Source: CAD feature listing. Evaluate the final solid. Frame: model axes, mm. A direction names the side the tool comes from. Round coordinates to 2 decimals unless told otherwise and drop trailing zeros. Loops run counter-clockwise (first coordinate to the right, second up) from the corner with the lowest first, then second, coordinate; pieces in that order, holes last.
(1) Section B-B, the plane x = -11.5. Return the cut outline in (y, z) (3 decimals).
(2) Set-up query: faces 4 (the cylindrical face through (-17.786, 5.966, 2.335)), 5 (the cylindrical face through (-3.36, 0.63, 9.82)). Return all of +Z, -Z, +X, -X, +Y, -Y with unobstructed straight access to the full face (end or side cutting, diameter ignored); none if empty.
(3) Section A-A, the plane z = -10. Return the cut outline in (x, y) (3 decimals).
(4) Mould query, pull axis Y, two halves, no side actions, for faces 1 (the cylindrical face through (-6.38, 5.95, 15.4)), 2 (the flat face through (0, 0, 0)), 3 (the flat face through (20, 1, 0)). Classes: pulls with the +Y half, pulls with the -Y half, needs draft (parallel to the pull), parting line crosses it, or undercut.
(5) Section D-D, the plane z = 15. Count the separate pieces of the cut face and the enclosed holes in it, plus the area to 3 significant figures.
(6) Section C-C, the plane y = 2.25. Return the cut outline in (x, z).
(7) Material intervals for probe 1 along Y at (x, z) = (-18, 7) (3 decimals); probe 2 along Z at (x, y) = (-5.5, 11.5); probe 3 along Z at (x, y) = (0.5, 6), sorted ascending.
```python
from build123d import *

# Parameters (mm, degrees)
SKETCH1_W           = 40
SKETCH1_H           = 40
SKETCH1_R           = 16.66875
SKETCH1_R_2         = 1.905
BOSS_EXTRUDE1_DEPTH = 1.27
SKETCH2_R           = 17.93875
SKETCH2_R_2         = 16.66875
BOSS_EXTRUDE2_DEPTH = 9.525
SKETCH3_W           = 40
SKETCH3_H           = 40
SKETCH3_R           = 16.66875
SKETCH3_R_2         = 1.905
BOSS_EXTRUDE3_DEPTH = 1.27
BOSS_EXTRUDE4_DEPTH = 1.27
BOSS_EXTRUDE5_START = -1.27
BOSS_EXTRUDE5_DEPTH = 1.27


with BuildPart() as part:
    # Sketch1 → Boss-Extrude1 (new body)
    with BuildSketch(Plane(origin=(0, 0, 0), x_dir=(1, 0, 0), z_dir=(0, 1, 0))):
        Rectangle(SKETCH1_W, SKETCH1_H)
        with Locations(Location((0, 0, 0), (0, 0, 270))):
            Circle(SKETCH1_R, mode=Mode.SUBTRACT)
        with Locations(Location((-15.875, 15.875, 0), (0, 0, 270))):
            Circle(SKETCH1_R_2, mode=Mode.SUBTRACT)
        with Locations(Location((15.875, 15.875, 0), (0, 0, 270))):
            Circle(SKETCH1_R_2, mode=Mode.SUBTRACT)
        with Locations(Location((-15.875, -15.875, 0), (0, 0, 270))):
            Circle(SKETCH1_R_2, mode=Mode.SUBTRACT)
        with Locations(Location((15.875, -15.875, 0), (0, 0, 270))):
            Circle(SKETCH1_R_2, mode=Mode.SUBTRACT)
    extrude(amount=BOSS_EXTRUDE1_DEPTH)

    # Sketch2 → Boss-Extrude2 (add)
    with BuildSketch(Plane(origin=(0, 1.27, 0), x_dir=(1, 0, 0), z_dir=(0, 1, 0))):
        with Locations(Location((0, 0, 0), (0, 0, 90))):
            Circle(SKETCH2_R)
        with Locations(Location((0, 0, 0), (0, 0, 270))):
            Circle(SKETCH2_R_2, mode=Mode.SUBTRACT)
    extrude(amount=BOSS_EXTRUDE2_DEPTH)

    # Sketch3 → Boss-Extrude3 (add)
    with BuildSketch(Plane(origin=(0, 10.795, 0), x_dir=(1, 0, 0), z_dir=(0, 1, 0))):
        Rectangle(SKETCH3_W, SKETCH3_H)
        with Locations(Location((0, 0, 0), (0, 0, 270))):
            Circle(SKETCH3_R, mode=Mode.SUBTRACT)
        with Locations(Location((-15.875, 15.875, 0), (0, 0, 270))):
            Circle(SKETCH3_R_2, mode=Mode.SUBTRACT)
        with Locations(Location((15.875, 15.875, 0), (0, 0, 270))):
            Circle(SKETCH3_R_2, mode=Mode.SUBTRACT)
        with Locations(Location((-15.875, -15.875, 0), (0, 0, 270))):
            Circle(SKETCH3_R_2, mode=Mode.SUBTRACT)
        with Locations(Location((15.875, -15.875, 0), (0, 0, 270))):
            Circle(SKETCH3_R_2, mode=Mode.SUBTRACT)
    extrude(amount=BOSS_EXTRUDE3_DEPTH)

    # Sketch4 → Boss-Extrude4 (add)
    with BuildSketch(Plane.XZ):
        with BuildLine():
            ThreePointArc((-1.922226487, 2.526988392), (-3.344814057, 9.921875), (0, 16.66875))
            ThreePointArc((0, 16.66875), (-4.314189958, 16.100776117), (-8.334375, 14.435560949))
            ThreePointArc((-8.334375, 14.435560949), (-6.829319423, 7.513884997), (-2.585941795, 1.84215364))
            ThreePointArc((-2.585941795, 1.84215364), (-3.079306216, 0.773626673), (-3.149549386, -0.401202774))
            ThreePointArc((-3.149549386, -0.401202774), (-10.265002832, 2.064243556), (-14.435560949, 8.334375))
            ThreePointArc((-14.435560949, 8.334375), (-16.100776117, 4.314189958), (-16.66875, 0))
            ThreePointArc((-16.66875, 0), (-9.921875, -2.157421613), (-2.888322747, -1.318414467))
            ThreePointArc((-2.888322747, -1.318414467), (-2.20963346, -2.279944073), (-1.227322899, -2.928191166))
            ThreePointArc((-1.227322899, -2.928191166), (-6.920188775, -7.857631444), (-14.435560949, -8.334375))
            ThreePointArc((-14.435560949, -8.334375), (-11.786586159, -11.786586159), (-8.334375, -14.435560949))
            ThreePointArc((-8.334375, -14.435560949), (-3.092555577, -9.67130661), (-0.302380952, -3.160568107))
            ThreePointArc((-0.302380952, -3.160568107), (0.869672756, -3.053570745), (1.922226487, -2.526988392))
            ThreePointArc((1.922226487, -2.526988392), (3.344814057, -9.921875), (0, -16.66875))
            ThreePointArc((0, -16.66875), (4.314189958, -16.100776117), (8.334375, -14.435560949))
            ThreePointArc((8.334375, -14.435560949), (6.829319423, -7.513884997), (2.585941795, -1.84215364))
            ThreePointArc((2.585941795, -1.84215364), (3.079306216, -0.773626673), (3.149549386, 0.401202774))
            ThreePointArc((3.149549386, 0.401202774), (10.265002832, -2.064243556), (14.435560949, -8.334375))
            ThreePointArc((14.435560949, -8.334375), (16.100776117, -4.314189958), (16.66875, 0))
            ThreePointArc((16.66875, 0), (9.921875, 2.157421613), (2.888322747, 1.318414467))
            ThreePointArc((2.888322747, 1.318414467), (2.20963346, 2.279944073), (1.227322899, 2.928191166))
            ThreePointArc((1.227322899, 2.928191166), (6.920188775, 7.857631444), (14.435560949, 8.334375))
            ThreePointArc((14.435560949, 8.334375), (11.786586159, 11.786586159), (8.334375, 14.435560949))
            ThreePointArc((8.334375, 14.435560949), (3.092555577, 9.67130661), (0.302380952, 3.160568107))
            ThreePointArc((0.302380952, 3.160568107), (-0.869672756, 3.053570745), (-1.922226487, 2.526988392))
        make_face()
    extrude(amount=-BOSS_EXTRUDE4_DEPTH)

    # Sketch5 → Boss-Extrude5 (add)
    with BuildSketch(Plane(origin=(0, 12.065, 0), x_dir=(1, 0, 0), z_dir=(0, 1, 0)).offset(BOSS_EXTRUDE5_START)):
        with BuildLine():
            ThreePointArc((1.227322899, -2.928191166), (6.920188775, -7.857631444), (14.435560949, -8.334375))
            ThreePointArc((14.435560949, -8.334375), (11.786586159, -11.786586159), (8.334375, -14.435560949))
            ThreePointArc((8.334375, -14.435560949), (3.092555577, -9.67130661), (0.302380952, -3.160568107))
            ThreePointArc((0.302380952, -3.160568107), (-0.869672756, -3.053570745), (-1.922226487, -2.526988392))
            ThreePointArc((-1.922226487, -2.526988392), (-3.344814057, -9.921875), (0, -16.66875))
            ThreePointArc((0, -16.66875), (-4.314189958, -16.100776117), (-8.334375, -14.435560949))
            ThreePointArc((-8.334375, -14.435560949), (-6.829319423, -7.513884997), (-2.585941795, -1.84215364))
            ThreePointArc((-2.585941795, -1.84215364), (-3.079306216, -0.773626673), (-3.149549386, 0.401202774))
            ThreePointArc((-3.149549386, 0.401202774), (-10.265002832, -2.064243556), (-14.435560949, -8.334375))
            ThreePointArc((-14.435560949, -8.334375), (-16.100776117, -4.314189958), (-16.66875, 0))
            ThreePointArc((-16.66875, 0), (-9.921875, 2.157421613), (-2.888322747, 1.318414467))
            ThreePointArc((-2.888322747, 1.318414467), (-2.20963346, 2.279944073), (-1.227322899, 2.928191166))
            ThreePointArc((-1.227322899, 2.928191166), (-6.920188775, 7.857631444), (-14.435560949, 8.334375))
            ThreePointArc((-14.435560949, 8.334375), (-11.786586159, 11.786586159), (-8.334375, 14.435560949))
            ThreePointArc((-8.334375, 14.435560949), (-3.092555577, 9.67130661), (-0.302380952, 3.160568107))
            ThreePointArc((-0.302380952, 3.160568107), (0.869672756, 3.053570745), (1.922226487, 2.526988392))
            ThreePointArc((1.922226487, 2.526988392), (3.344814057, 9.921875), (0, 16.66875))
            ThreePointArc((0, 16.66875), (4.314189958, 16.100776117), (8.334375, 14.435560949))
            ThreePointArc((8.334375, 14.435560949), (6.829319423, 7.513884997), (2.585941795, 1.84215364))
            ThreePointArc((2.585941795, 1.84215364), (3.079306216, 0.773626673), (3.149549386, -0.401202774))
            ThreePointArc((3.149549386, -0.401202774), (10.265002832, 2.064243556), (14.435560949, 8.334375))
            ThreePointArc((14.435560949, 8.334375), (16.100776117, 4.314189958), (16.66875, 0))
            ThreePointArc((16.66875, 0), (9.921875, -2.157421613), (2.888322747, -1.318414467))
            ThreePointArc((2.888322747, -1.318414467), (2.20963346, -2.279944073), (1.227322899, -2.928191166))
        make_face()
    extrude(amount=BOSS_EXTRUDE5_DEPTH)


solid = part.part
```
Output values:
1. outline: (0, -20) - (1.27, -20) - (1.27, -13.768) - (10.795, -13.768) - (10.795, -20) - (12.065, -20) - (12.065, -8.735) - (10.795, -8.735) - (10.795, -12.066) - (1.27, -12.066) - (1.27, -8.735) - (0, -8.735) - close; (0, -1.93) - (1.27, -1.93) - (1.27, 3.167) - (0, 3.167) - close; (0, 12.066) - (12.065, 12.066) - (12.065, 20) - (10.795, 20) - (10.795, 13.768) - (1.27, 13.768) - (1.27, 20) - (0, 20) - close; (10.795, -1.93) - (12.065, -1.93) - (12.065, 3.167) - (10.795, 3.167) - close
2. face 4: none
2. face 5: +Y, -Y
3. outline: (-20, 0) - (-3.333, 0) - (-3.333, 1.27) - (-13.336, 1.27) - (-13.336, 10.795) - (-3.333, 10.795) - (-3.333, 12.065) - (-20, 12.065) - (-20, 10.795) - (-14.893, 10.795) - (-14.893, 1.27) - (-20, 1.27) - close; (3.334, 0) - (7.733, 0) - (7.733, 1.27) - (3.334, 1.27) - close; (3.334, 10.795) - (7.733, 10.795) - (7.733, 12.065) - (3.334, 12.065) - close; (13.336, 0) - (20, 0) - (20, 1.27) - (14.893, 1.27) - (14.893, 10.795) - (20, 10.795) - (20, 12.065) - (13.336, 12.065) - close
4. face 1: undercut
4. face 2: pulls with the -Y half
4. face 3: needs draft
5. separate pieces: 6
5. enclosed holes: 0
5. area: 111 mm2
6. outline: circle Ø35.88 at (0, 0); hole circle Ø33.34 at (0, 0)
7. probe 1: y = 0 to 1.27, 10.795 to 12.065
7. probe 2: z = -20 to -15.74, -12.37 to -7.16, -1.99 to -0.14, 5.14 to 20
7. probe 3: z = -17.93 to -16.66, 16.66 to 17.93
